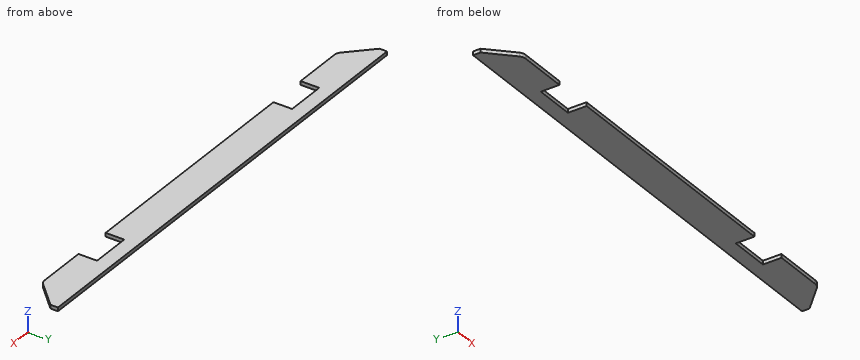
from build123d import *

# Parameters (mm, degrees)
BOSS_EXTRUDE1_DEPTH = 3


with BuildPart() as part:
    # Sketch1 → Boss-Extrude1 (new body)
    with BuildSketch(Plane.XY):
        with BuildLine():
            Line((130.955345629, -26.5), (170.433838397, -26.5))
            ThreePointArc((170.433838397, -26.5), (173.093720589, -26.044378238), (175.383585865, -24.616414135))
            Line((175.383585865, -24.616414135), (194, -6))
            Line((194, -6), (194, 0))
            Line((194, 0), (-194, 0))
            Line((-194, 0), (-194, -6))
            Line((-194, -6), (-175.383585865, -24.616414135))
            ThreePointArc((-175.383585865, -24.616414135), (-173.093720589, -26.044378238), (-170.433838397, -26.5))
            Line((-170.433838397, -26.5), (-130.955345629, -26.5))
            Line((-130.955345629, -26.5), (-130.955345629, -11.5))
            Line((-130.955345629, -11.5), (-98.955345629, -11.5))
            Line((-98.955345629, -11.5), (-98.955345629, -26.5))
            Line((-98.955345629, -26.5), (98.955345629, -26.5))
            Line((98.955345629, -26.5), (98.955345629, -11.5))
            Line((98.955345629, -11.5), (130.955345629, -11.5))
            Line((130.955345629, -11.5), (130.955345629, -26.5))
        make_face()
    extrude(amount=BOSS_EXTRUDE1_DEPTH)


solid = part.part
Part model, mm, in its own coordinate system. Round coordinates to 2 decimals unless told otherwise and drop trailing zeros. Write each loop counter-clockwise with the first axis right and the second up, starting at its lowest first coordinate (ties: lowest second). Pieces come first, ordered by that corner, then holes. Notation, with made-up numbers: M 16,-40 L 30,-40 A37 ccw 30,-2 Z; hole C -20.75,-9.75 d7. An arc over 180 degrees is marked long. Return JSON: item names as keys, results as strings. Group by question number.
(1) Drill centre lines: probe 1 along X at (y, z) = (-17.25, 0.9); probe 2 along X at (y, z) = (-23.25, 1.5); probe 3 along Y at (x, z) = (-96.5, 1.6). Where is each one in solid material? Low to high.
(2) Saw through at A-A on y = -19.5. Write the cut outline in (x, z), then the cut area to 3 significant figures.
(3) Saw through at C-C on x = 104. Write the cut outline in (y, z).
(4) Pin check, flat tips, straight feed: pin 1 Ø1.5 at (y, z) = (-18, 1) entering from +X; pin 2 Ø0.9 at (y, z) = (-18, 1.5) entering from -X; pin 3 Ø1 at (y, z) = (-23, 0.5) entering from +X. Stop position of each tip, or through.
(5) Saw through at B-B on z = 0.95. Write the cut outline in (x, y).
Returned:
{
 "1": {"probe 1": "-182.75 to -130.96, -98.96 to 98.96, 130.96 to 182.75", "probe 2": "-176.75 to -130.96, -98.96 to 98.96, 130.96 to 176.75", "probe 3": "-26.5 to 0"},
 "2": {"outline": "M -180.5,0 L -130.96,0 L -130.96,3 L -180.5,3 Z; M -98.96,0 L 98.96,0 L 98.96,3 L -98.96,3 Z; M 130.96,0 L 180.5,0 L 180.5,3 L 130.96,3 Z", "area": "891 mm²"},
 "3": {"outline": "M -11.5,0 L 0,0 L 0,3 L -11.5,3 Z"},
 "4": {"pin 1": "x = 182.75", "pin 2": "x = -182.45", "pin 3": "x = 177.5"},
 "5": {"outline": "M -194,-6 L -175.38,-24.62 A7 ccw -170.43,-26.5 L -130.96,-26.5 L -130.96,-11.5 L -98.96,-11.5 L -98.96,-26.5 L 98.96,-26.5 L 98.96,-11.5 L 130.96,-11.5 L 130.96,-26.5 L 170.43,-26.5 A7 ccw 175.38,-24.62 L 194,-6 L 194,0 L -194,0 Z"}
}
